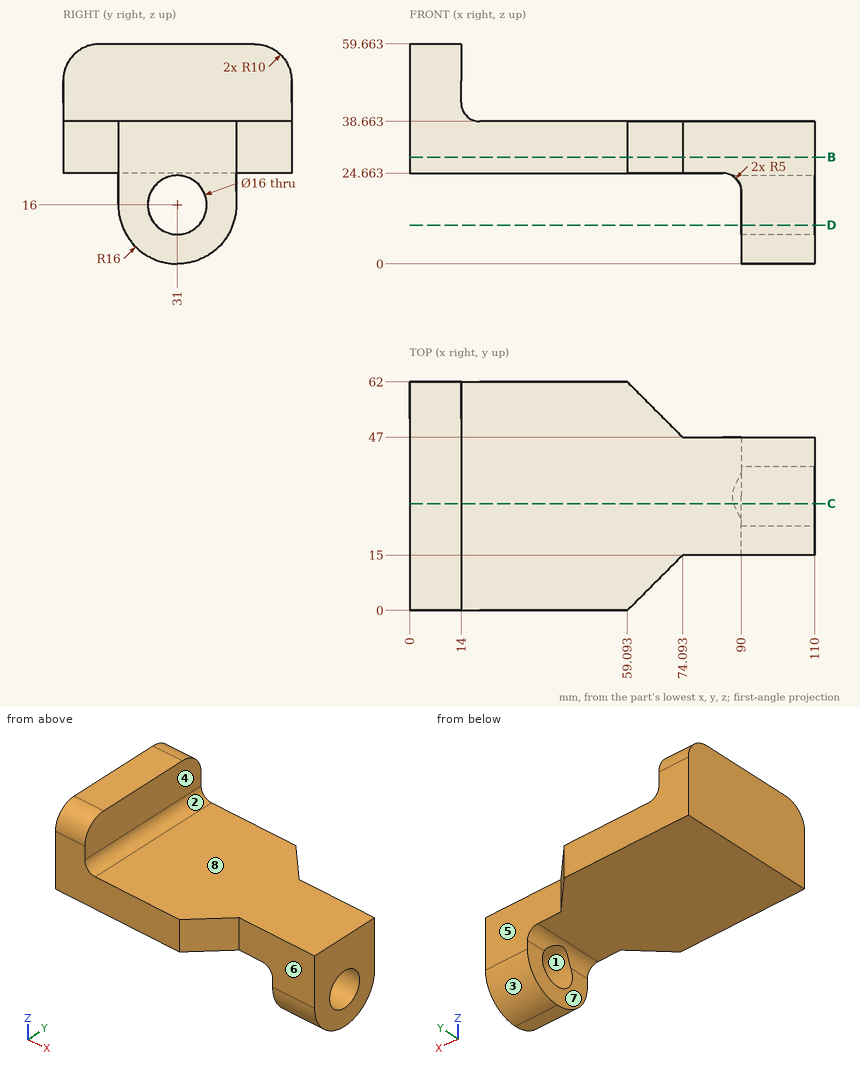
Geometry: see drawing. Coordinates: mm, zero at the bounding-box minimum. A direction names the side the tool comes from. Round coordinates to 2 decimals unless told otherwise and drop trailing zeros. Loops run counter-clockwise (first coordinate to the right, second up) from the corner with the lowest first, then second, coordinate; pieces in that order, holes last. Notation, with made-up numbers: (29.25, 7) -> (60.25, 7) arc R24 ccw to (60.25, 30) -> close; hole circle Ø11 at (-5.75, 75.5). An arc over 180 degrees is marked (long way). Write each question's results on one line, items separated by ' | '.
1. First-contact query: P1, Ø6, axis at y = 32.5, z = 12.5, coming from the -X side; P2, Ø25, axis at x = 91, z = 30, coming from the -Y side; P3, Ø3, axis at x = 58, y = 42, coming from the +Z side; P4, Ø5, axis at y = 34, z = 55.5, coming from the +X side. Flat tips, straight axial feed; report the tip coordinate or a pass-through.
Geometry results:
P1: through | P2: y = 15 | P3: z = 38.66 | P4: x = 14
2. Section D-D (z = 10.5). Return loops of the section in (x, y) (1 decimal).
Geometry results:
outline: (90, 16) -> (110, 16) -> (110, 25.2) -> (90, 25.2) -> close; (90, 36.8) -> (110, 36.8) -> (110, 46) -> (90, 46) -> close
3. Section C-C (y = 29). Return loops of the section in (x, z).
Geometry results:
outline: (0, 24.66) -> (85, 24.66) arc R5 cw to (87.89, 23.75) -> (110, 23.75) -> (110, 38.66) -> (19, 38.66) arc R5 cw to (14, 43.66) -> (14, 59.66) -> (0, 59.66) -> close; (90, 0.13) -> (110, 0.13) -> (110, 8.25) -> (90, 8.25) -> close
4. Ray query, line 1 (Z direction, x = 101, y = 31); line 2 (X direction, y = 56.5, z = 52.5); line 3 (Z direction, x = 30.5, y = 44). Return the intervals inside material, ascending. Write a range as from..to.
Geometry results:
line 1: 0..8, 24..38.66 | line 2: 0..14 | line 3: 24.66..38.66
5. Section B-B (z = 29). Return loops of the section in (x, y).
Geometry results:
outline: (0, 0) -> (59.09, 0) -> (74.09, 15) -> (110, 15) -> (110, 47) -> (74.09, 47) -> (59.09, 62) -> (0, 62) -> close
6. Set-up query: the marked faces 5, 6, 7 and 8. Return all of +Z, -Z, +X, -X, +Y, -Y with unobstructed straight access to the full face (end or side cutting, diameter ignored); none if empty.
Geometry results:
face 5: +Z, -Z, +X, +Y | face 6: +Z, -Z, +X, -Y | face 7: -Z, -X, +Y, -Y | face 8: +Z, +X, +Y, -Y
7. Mould query, pull axis Z, two halves, no side actions, for the marked faces 1, 2, 3 and 4. Classes: +Z half, -Z half, draft (parallel to the pull), parting line (faces both ways), or undercut.
Geometry results:
face 1: undercut | face 2: +Z half | face 3: -Z half | face 4: draft
